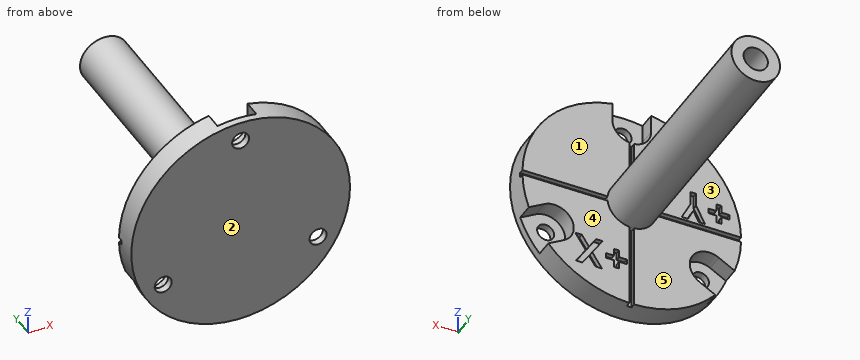
```python
from build123d import *

# Parameters (mm, degrees)
SKETCH1_R                = 22.5
PLATE_DEPTH              = 5
OPENING_START            = 1.5
OPENING_FOR_SCREW_DEPTH  = 5
SKETCH7_R                = 1.75
SCREW_HOLE_DEPTH         = 5
CIRPATTERN20_COUNT       = 3
SKETCH10_W               = 45
SKETCH10_H               = 1
SKETCH10_W_2             = 1
SKETCH10_H_2             = 45
CUT_EXTRUDE5_DEPTH       = 1
CUT_EXTRUDE6_DEPTH       = 1
SKETCH12_R               = 5
SKETCH12_R_2             = 2.5
BOSS_EXTRUDE2_DEPTH      = 50
BOSS_EXTRUDE2_DEPTH_BACK = 1


with BuildPart() as part:
    # Sketch1 → plate (new body)
    with BuildSketch(Plane(origin=(0, 0, 0), x_dir=(1, 0, 0), z_dir=(0, 1, 0))):
        Circle(SKETCH1_R)
    extrude(amount=PLATE_DEPTH)

    # Sketch6 → opening for screw (cut)
    with BuildSketch(Plane(origin=(0, 5, 0), x_dir=(1, 0, 0), z_dir=(0, 1, 0)).offset(OPENING_START)):
        with BuildLine():
            Line((-4, -22.5), (-4, -18.4))
            ThreePointArc((-4, -18.4), (0, -14.4), (4, -18.4))
            Line((4, -18.4), (4, -22.5))
            ThreePointArc((4, -22.5), (0, -26.5), (-4, -22.5))
        make_face()
    opening_for_screw = extrude(amount=-OPENING_FOR_SCREW_DEPTH, mode=Mode.SUBTRACT)

    # Sketch7 → screw hole (cut)
    with BuildSketch(Plane(origin=(0, 1.5, 0), x_dir=(1, 0, 0), z_dir=(0, 1, 0))):
        with Locations((0, -18.4)):
            Circle(SKETCH7_R)
    screw_hole = extrude(amount=-SCREW_HOLE_DEPTH, mode=Mode.SUBTRACT)

    # CirPattern20: opening for screw, screw hole ×3 about axis
    cirpattern20_axis = Axis((0, 0, 0), (0, 1, 0))
    for i in range(1, CIRPATTERN20_COUNT):
        add(opening_for_screw.rotate(cirpattern20_axis, i * 360 / CIRPATTERN20_COUNT), mode=Mode.SUBTRACT)
        add(screw_hole.rotate(cirpattern20_axis, i * 360 / CIRPATTERN20_COUNT), mode=Mode.SUBTRACT)

    # Sketch10 → Cut-Extrude5 (cut)
    with BuildSketch(Plane(origin=(0, 5, 0), x_dir=(1, 0, 0), z_dir=(0, 1, 0))):
        Rectangle(SKETCH10_W, SKETCH10_H)
        Rectangle(SKETCH10_W_2, SKETCH10_H_2)
    extrude(amount=-CUT_EXTRUDE5_DEPTH, mode=Mode.SUBTRACT)

    # Sketch11 → Cut-Extrude6 (cut)
    with BuildSketch(Plane(origin=(0, 5, 0), x_dir=(1, 0, 0), z_dir=(0, 1, 0))):
        Polygon((2.616666667, 13.742425761), (2.616666667, 15.289220632), (3.675, 15.289220632), (3.675, 13.742425761), (5.303205128, 13.742425761), (5.303205128, 12.684092427), (3.675, 12.684092427), (3.675, 11.137297556), (2.616666667, 11.137297556), (2.616666667, 12.684092427), (0.988461538, 12.684092427), (0.988461538, 13.742425761), align=None)
        Polygon((6.136388221, 16.510374479), (7.479657452, 16.510374479), (8.806390224, 14.471301963), (10.135667067, 16.510374479), (11.480208333, 16.510374479), (9.47802484, 13.43968137), (11.6125, 10.160374479), (10.269230769, 10.160374479), (8.806390224, 12.409332812), (7.339733574, 10.160374479), (5.995192308, 10.160374479), (8.134755609, 13.440953405), align=None)
        Polygon((-18.458103671, -3.794817635), (-18.458103671, -2.248022763), (-17.399770338, -2.248022763), (-17.399770338, -3.794817635), (-15.771565209, -3.794817635), (-15.771565209, -4.853150968), (-17.399770338, -4.853150968), (-17.399770338, -6.39994584), (-18.458103671, -6.39994584), (-18.458103671, -4.853150968), (-20.086308799, -4.853150968), (-20.086308799, -3.794817635), align=None)
        Polygon((-15.07957803, -1.026868917), (-13.811358879, -1.026868917), (-12.677975466, -3.254202651), (-11.544592052, -1.026868917), (-10.276372902, -1.026868917), (-12.108103671, -4.626728693), (-12.108103671, -7.376868917), (-13.247847261, -7.376868917), (-13.247847261, -4.626728693), align=None)
    extrude(amount=-CUT_EXTRUDE6_DEPTH, mode=Mode.SUBTRACT)

    # Sketch12 → Boss-Extrude2 (add, two sides)
    with BuildSketch(Plane(origin=(0, 5, 0), x_dir=(1, 0, 0), z_dir=(0, 1, 0))) as boss_extrude2_sk:
        Circle(SKETCH12_R)
        Circle(SKETCH12_R_2, mode=Mode.SUBTRACT)
    extrude(amount=BOSS_EXTRUDE2_DEPTH)
    extrude(boss_extrude2_sk.sketch, amount=-BOSS_EXTRUDE2_DEPTH_BACK)


solid = part.part
```
Build history of the part. All positions in model axes, mm. Face numbers are marked on the shaded views. A direction names the side the tool comes from. Coordinates: 2 decimals unless noted, no trailing zeros. Write each loop counter-clockwise with the first axis right and the second up, starting at its lowest first coordinate (ties: lowest second). Pieces come first, ordered by that corner, then holes.
1. Band-saw the part on A-A, the plane z = -9.2. Give the cut face in (x, y).
Answer block:
outline: (-20.53, 0) - (-17.68, 0) - (-17.68, 1.5) - (-20.53, 1.5) - close; (-14.18, 0) - (14.18, 0) - (14.18, 1.5) - (11.93, 1.5) - (11.93, 5) - (0.5, 5) - (0.5, 4) - (-0.5, 4) - (-0.5, 5) - (-11.93, 5) - (-11.93, 1.5) - (-14.18, 1.5) - close; (17.68, 0) - (20.53, 0) - (20.53, 1.5) - (17.68, 1.5) - close
2. Band-saw the part on B-B, the plane x = -8.5. Give the cut face in (y, z).
Answer block:
outline: (0, -20.83) - (5, -20.83) - (5, -0.5) - (4, -0.5) - (4, 0.5) - (5, 0.5) - (5, 20.83) - (0, 20.83) - close
3. Band-saw the part on D-D, the plane z = 11.5. Give the cut face in (x, y), and give its area (3 significant figures).
Answer block:
outline: (-19.34, 0) - (19.34, 0) - (19.34, 5) - (0.5, 5) - (0.5, 4) - (-0.5, 4) - (-0.5, 5) - (-19.34, 5) - close
area: 192 mm2
4. Drill centre lines: probe 1 along Y at (x, z) = (-19.5, -8); probe 2 along Y at (x, z) = (13, -14); probe 3 along Z at (x, y) = (0.5, 34). Where is each one in solid material? Low to high.
Answer block:
probe 1: y = 0 to 1.5
probe 2: y = 0 to 5
probe 3: z = -4.97 to -2.45, 2.45 to 4.97
5. Band-saw the part on C-C, the plane y = 18.5. Give the cut face in (x, z).
Answer block:
outline: circle Ø10 at (0, 0); hole circle Ø5 at (0, 0)
6. 3-axis set-ups, long thin cutter, end or side, ignore diameter. For the marked faces 1, 2, 3, 4 and 5: which of +Z, -Z, +X, -X, +Y, -Y reach the whole face in a straight line?
Answer block:
face 1: +Z, +X, +Y
face 2: +Z, -Z, +X, -X, -Y
face 3: +Z, -X, +Y
face 4: -Z, +X, +Y
face 5: -Z, -X, +Y
7. Drop flat-ended pins along their axis: pin 1 (2 mm diameter, centred on x = -5.5, z = 4.5, fed in from +Y); pin 2 (0.5 mm diameter, centred on y = 4.5, z = 5.5, fed in from +X); pin 3 (12 mm diameter, centred on y = 17, z = -4.5, fed in from -X). Give the stop position or say it passes through.
Answer block:
pin 1: stops at y = 5
pin 2: stops at x = 21.88
pin 3: stops at x = -5
